Model file for the job. Use its own axes, mm. A direction names the side the tool comes from. Round coordinates to 2 decimals unless told otherwise and drop trailing zeros. Write each loop counter-clockwise with the first axis right and the second up, starting at its lowest first coordinate (ties: lowest second). Pieces come first, ordered by that corner, then holes. Notation, with made-up numbers: (77, 88) - (83, 88) arc R9 ccw to (83, 103) - close; hole circle Ø3 at (49.25, 6.25). An arc over 180 degrees is marked (long way). One line per item, written item: value.
from build123d import *

# Parameters (mm, degrees)
F0_W     = 35
F0_H     = 10
F1_DEPTH = 10
F2_R     = 2


# Not quite as in the source:
# - a feature names something its author has since deleted; it is built from what else it names


with BuildPart() as f1:
    # F0 (on Top) → F1 (new body)
    with BuildSketch(Plane.XY):
        Rectangle(F0_W, F0_H)
        with BuildLine():
            Line((-8, 1.5), (0, 1.5))
            Line((0, 1.5), (8, 1.5))
            ThreePointArc((8, 1.5), (9.5, 0), (8, -1.5))
            Line((8, -1.5), (0, -1.5))
            Line((0, -1.5), (-8, -1.5))
            ThreePointArc((-8, -1.5), (-9.5, 0), (-8, 1.5))
        make_face(mode=Mode.SUBTRACT)
        Polygon((17.5, 15), (17.5, 5), (17.5, -5), (17.5, -15), (27.5, -15), (27.5, 15), align=None)
        with BuildLine():
            ThreePointArc((27.5, -15), (42.5, 0), (27.5, 15))
            Line((27.5, 15), (27.5, -15))
        make_face()
    extrude(amount=F1_DEPTH)

    # F2
    f2_edges = [f1.edges().sort_by_distance(p)[0] for p in [
        (27.5, 15, 5),
        (27.5, -15, 5),
        (42.5, 0, 10),
        (42.5, 0, 0),
        (17.5, 10, 10),
        (17.5, -10, 10),
        (17.5, -15, 5),
        (17.5, 10, 0),
        (17.5, -10, 0),
        (17.5, 15, 5),
    ]]
    fillet(f2_edges, radius=F2_R)


solid = f1.part
1. Wall check: probe 1 along Y at (x, z) = (3.5, 8.75); probe 2 along Y at (x, z) = (-11, 5.5); probe 3 along Y at (x, z) = (8.5, 8.5). Give the ranges that are in metal, low to high. Write a range as [from, to].
Report:
probe 1: [-5, -1.5], [1.5, 5]
probe 2: [-5, 5]
probe 3: [-5, -1.41], [1.41, 5]
2. Band-saw the part on A-A on y = 0. Write the cut outline in (x, z).
Report:
outline: (-17.5, 0) - (-9.5, 0) - (-9.5, 10) - (-17.5, 10) - close; (9.5, 0) - (40.5, 0) arc R2 ccw to (42.5, 2) - (42.5, 8) arc R2 ccw to (40.5, 10) - (9.5, 10) - close
3. Band-saw the part on C-C on x = -5. Write the cut outline in (y, z), plus the area to 3 significant figures.
Report:
outline: (-5, 0) - (-1.5, 0) - (-1.5, 10) - (-5, 10) - close; (1.5, 0) - (5, 0) - (5, 10) - (1.5, 10) - close
area: 70.0 mm²
4. Drop flat-ended pins along their axis: pin 1 (1.8 mm diameter, centred on y = 8.5, z = 6.5, fed in from -X); pin 2 (4 mm diameter, centred on x = 1.5, z = 5.5, fed in from +Y). Give the stop position or say it passes through.
Report:
pin 1: x = 17.5
pin 2: y = 5
5. Mould opens along Y. For faces 6 (the face through (-9.5, 0, 4.9)), 7 (the face through (1, -5, 5)), 8 (the face through (23.44, 14.43, 0.6)), 9 (the face through (18, 0, 0)) say: released by +Y, released by -Y, zero draft, split by the parting line, or undercut.
Report:
face 6: undercut
face 7: released by -Y
face 8: released by +Y
face 9: zero draft
6. Tool access for faces 1 (the face through (0, 1.5, 5)), 2 (the face through (18.07, 8.94, 9.4)), 3 (the face through (17.5, 9, 5)), 4 (the face through (17.5, -9, 5)), 5 (the face through (18.07, 8.94, 0.6)): list every direction of +Z, -Z, +X, -X, +Y, -Y with a clear straight run to the whole face (end or side of a thin tool).
Report:
face 1: +Z, -Z
face 2: +Z, -X, +Y
face 3: +Z, -Z, -X, +Y
face 4: +Z, -Z, -X, -Y
face 5: -Z, -X, +Y
7. Band-saw the part on D-D on x = 18.5. Write the cut outline in (y, z), plus the area to 3 significant figures.
Report:
outline: (-14.73, 2) arc R1.73 ccw to (-13, 0.27) - (-5, 0.27) - (-5, 0) - (5, 0) - (5, 0.27) - (13, 0.27) arc R1.73 ccw to (14.73, 2) - (14.73, 8) arc R1.73 ccw to (13, 9.73) - (5, 9.73) - (5, 10) - (-5, 10) - (-5, 9.73) - (-13, 9.73) arc R1.73 ccw to (-14.73, 8) - close
area: 282 mm²
8. Band-saw the part on B-B on z = 3.25. Write the cut outline in (x, y).
Report:
outline: (-17.5, -5) - (17.5, -5) - (17.5, -13) arc R2 ccw to (19.5, -15) - (27.5, -15) arc R15 ccw to (27.5, 15) - (19.5, 15) arc R2 ccw to (17.5, 13) - (17.5, 5) - (-17.5, 5) - close; hole (-8, -1.5) - (8, -1.5) arc R1.5 ccw to (8, 1.5) - (-8, 1.5) arc R1.5 ccw to start
